Part print with two shaded views. Sizes in mm from the minimum x, y, z corner. A direction names the side the tool comes from. Coordinates: 2 decimals unless noted, no trailing zeros. Loops run counter-clockwise (first coordinate to the right, second up) from the corner with the lowest first, then second, coordinate; pieces in that order, holes last.
Item 1: Flat gauge pins, fed straight in: pin 1 (5 mm diameter, centred on x = 11, z = 8, fed in from +Y); pin 2 (11 mm diameter, centred on x = 40, y = 34, fed in from -Z); pin 3 (3 mm diameter, centred on y = 29.5, z = 2.5, fed in from -X); pin 4 (5 mm diameter, centred on x = 50, z = 3, fed in from +Y). Where does each tip first touch, or does it go through?
Item 2: Cut at C-C (y = 32). List the corners of the cut face in (x, z), and give its area (3 significant figures).
Item 3: Drill centre lines: line 1 along X through (y, z) = (3.8, 6.5); line 2 along X through (y, z) = (34, 9.25); line 3 along X through (y, z) = (10.5, 9.5). Where is each one in solid material? Low to high.
Item 4: 3-axis set-ups, long thin cutter, end or side, ignore diameter. For the marked faces 1, 2, 3, 4 and 5: which of +Z, -Z, +X, -X, +Y, -Y reach the whole face in a straight line?
Item 5: Cut at B-B (z = 6.5). Count the separate pieces of the cut face and the enclosed holes in it, and give its area (3 significant figures).
Item 6: Cut at D-D (x = 70). List the corners of the cut face in (y, z), and give its area (3 significant figures).
Item 7: Cut at A-A (x = 40). List the corners of the cut face in (y, z).
Item 8: Mould opens along Z. For the marked faces 6, 7 and 8 say: released by +Z, released by -Z, zero draft, split by the parting line, or undercut.
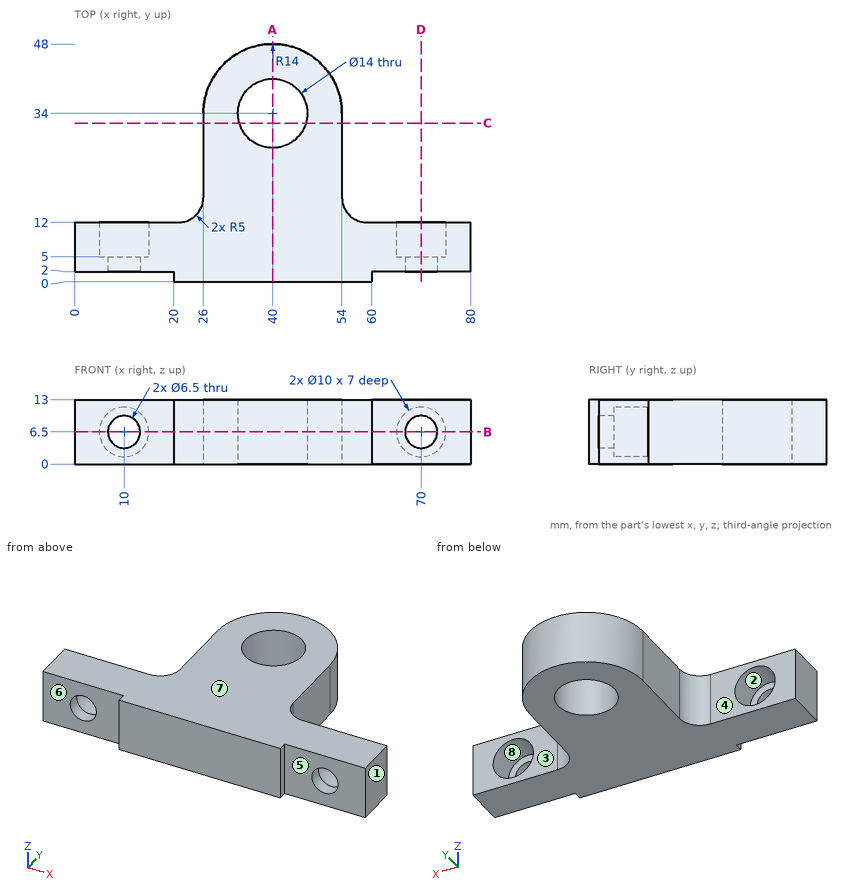
Filled sheet:
1. pin 1: stops at y = 5
1. pin 2: passes through
1. pin 3: stops at x = 26
1. pin 4: stops at y = 45.82
2. outline: (26, 0) - (33.29, 0) - (33.29, 13) - (26, 13) - close; (46.71, 0) - (54, 0) - (54, 13) - (46.71, 13) - close
2. area: 190 mm2
3. line 1: x = 0 to 6.75, 13.25 to 66.75, 73.25 to 80
3. line 2: x = 26 to 33, 47 to 54
3. line 3: x = 0 to 6, 14 to 66, 74 to 80
4. face 1: +Z, -Z, +X, +Y, -Y
4. face 2: +Y
4. face 3: +Z, -Z, +X, +Y
4. face 4: +Z, -Z, -X, +Y
4. face 5: +Z, -Z, +X, -Y
5. separate pieces: 3
5. enclosed holes: 1
5. area: 1,480 mm2
6. outline: (2, 0) - (12, 0) - (12, 1.5) - (5, 1.5) - (5, 3.25) - (2, 3.25) - close; (2, 9.75) - (5, 9.75) - (5, 11.5) - (12, 11.5) - (12, 13) - (2, 13) - close
6. area: 40.5 mm2
7. outline: (0, 0) - (27, 0) - (27, 13) - (0, 13) - close; (41, 0) - (48, 0) - (48, 13) - (41, 13) - close
8. face 6: zero draft
8. face 7: released by +Z
8. face 8: undercut
